Could you check a few things on this drawing? It's one solid part, dimensions in mm from its lowest x, y, z. Coordinates: 2 decimals unless noted, no trailing zeros. Loops run counter-clockwise (first coordinate to the right, second up) from the corner with the lowest first, then second, coordinate; pieces in that order, holes last. Notation, with made-up numbers: M -12.5,6.25 L 32.5,6.25 A11 cw 32.5,19.25 Z; hole C 48.5,16.5 d6. An arc over 180 degrees is marked long. Use one line per item in the form item = value. Start each with the question number.
(1) Imagine slicing it at B-B, the plane z = 12. Please give me the cut outline in (x, y), and give its area (3 significant figures).
(2) Will these pins go through, and if not, where does the flat tip stop? P1, Ø7, axis at x = 11.5, z = 16.5, coming from the -Y side; P2, Ø10, axis at y = 11, z = 19.5, coming from the -X side; P3, Ø1, axis at x = 20.5, y = 14, coming from the +Z side.
(3) Imagine slicing it at A-A, the plane x = 12. Please give me the cut outline in (y, z).
(4) Imagine slicing it at C-C, the plane y = 26. Please give me the cut outline in (x, z).
(5) Please list where these lines run through material, in increasing order: L1, parallel to Y at x = 19.75, z = 15.25; L2, parallel to Z at x = 20.5, y = 13.7; L3, parallel to Z at x = 11.5, y = 45.
(6) Imagine slicing it at D-D, the plane x = 20.5. Please give me the cut outline in (y, z).
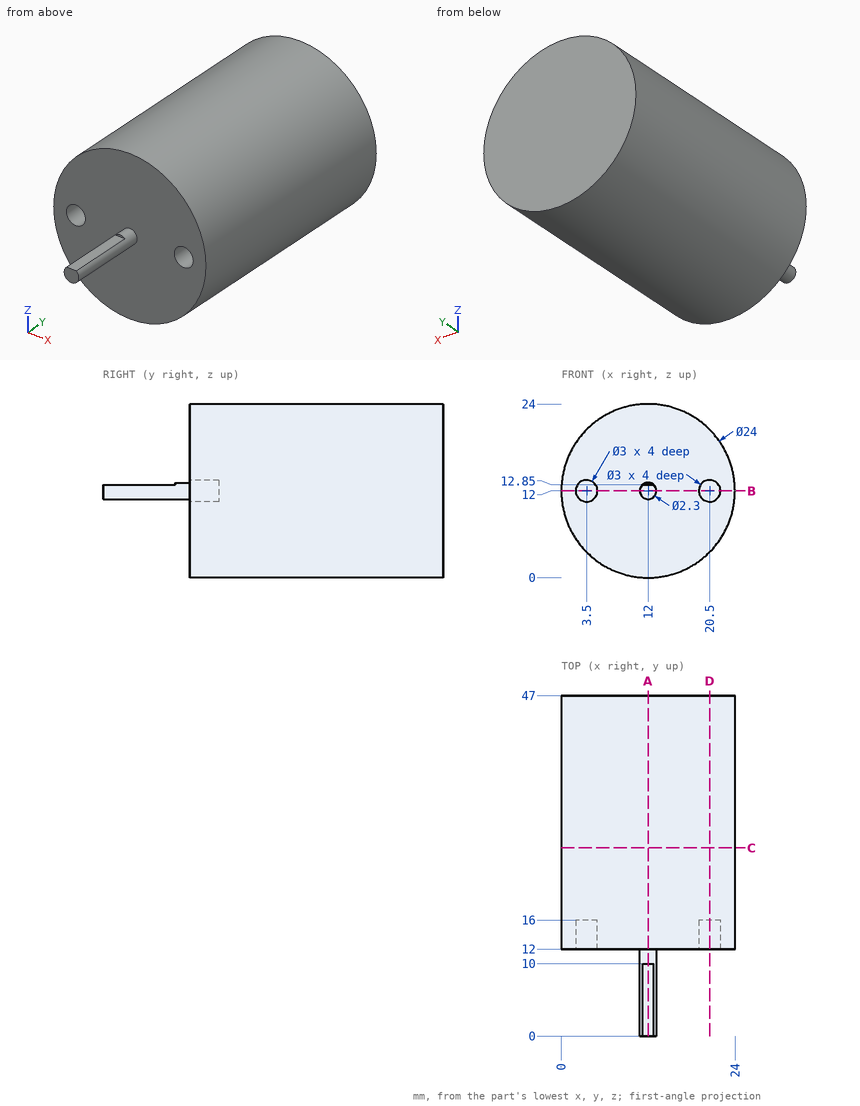
Answer:
q1.outline = M 0,12 L 2,12 L 2,16 L 5,16 L 5,12 L 10.85,12 L 10.85,0 L 13.15,0 L 13.15,12 L 19,12 L 19,16 L 22,16 L 22,12 L 24,12 L 24,47 L 0,47 Z
q1.area = 844 mm²
q2.P1 = 10
q2.P2 = 0.29
q2.P3 = 20.94
q3.outline = M 0,10.85 L 12,10.85 L 12,0 L 47,0 L 47,24 L 12,24 L 12,13.15 L 10,13.15 L 10,12.85 L 0,12.85 Z
q4.outline = C 12,12 d24
q5.L1 = 12 to 47
q5.L2 = 3.53 to 10.5, 13.5 to 20.47
q5.L3 = 0.01 to 23.99
q6.outline = M 12,3.53 L 47,3.53 L 47,20.47 L 12,20.47 L 12,13.5 L 16,13.5 L 16,10.5 L 12,10.5 Z
